For this review, use the dimensioned drawing (mm, ordinates from the lowest corner) and the shaded views. A direction names the side the tool comes from. Give positions to 0.01 mm unless a question says otherwise; leave off trailing zeros. Write each loop counter-clockwise with the first axis right and the second up, starting at its lowest first coordinate (ties: lowest second). Pieces come first, ordered by that corner, then holes. Notation, with made-up numbers: M 45.25,76 L 55.25,76 A22 ccw 55.25,95 Z; hole C -1.5,73.25 d6. An arc over 180 degrees is marked long. One line per item, written item: value. Start each with the question number.
Item 1: Tool access review of the marked faces 1 and 2: name each direction out of +Z, -Z, +X, -X, +Y, -Y from which nothing blocks a thin tool from reaching the whole face with its end or side.
Item 2: Mouldability with a two-part tool opening along X and no side actions: class the marked faces 3, 4 and 5 as released by +X, released by -X, zero draft, split by the parting line, or undercut.
Item 3: Consider section D-D, the plane x = 64.5. Write out the cut boundary in (y, z).
Item 4: Consider section B-B, the plane y = 37.5. Write out the cut boundary in (x, z).
Item 5: Consider section C-C, the plane z = 23. Write out the cut boundary in (x, y), and give its area (3 significant figures).
Item 6: Consider section A-A, the plane x = 39. Write out the cut boundary in (y, z), and give its area (3 significant figures).
Item 7: To check wall thickness, follow probe 1 along X at (y, z) = (17, 9); probe 2 along Z at (x, y) = (64.5, 27.1); probe 3 along Y at (x, z) = (53.5, 16). State the ranges of each line that lie inside material, in increasing order.
Item 8: Clearance check with flat-ended pins moving along their axes: pin 1 Ø3.5 at (x, z) = (64.5, 37) entering from +Y; pin 2 Ø5 at (x, z) = (64.5, 9) entering from -Y; pin 3 Ø0.9 at (x, y) = (36.5, 17.5) entering from -Z. State where each tip first meets the part, or that it passes through.
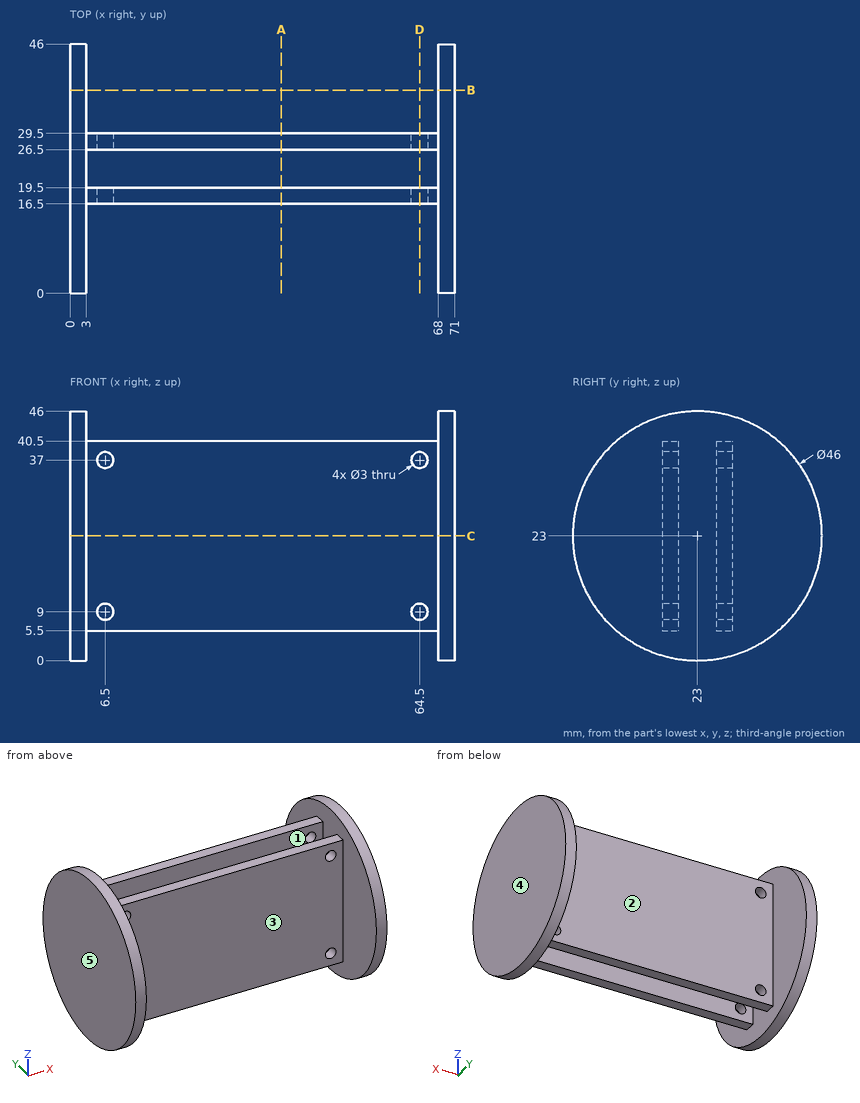
Model answer:
1. face 1: +Z, -Z
1. face 2: +Z, -Z, +Y
2. face 3: undercut
2. face 4: released by +X
2. face 5: released by -X
3. outline: M 16.5,5.5 L 19.5,5.5 L 19.5,7.5 L 16.5,7.5 Z; M 16.5,10.5 L 19.5,10.5 L 19.5,35.5 L 16.5,35.5 Z; M 16.5,38.5 L 19.5,38.5 L 19.5,40.5 L 16.5,40.5 Z; M 26.5,5.5 L 29.5,5.5 L 29.5,7.5 L 26.5,7.5 Z; M 26.5,10.5 L 29.5,10.5 L 29.5,35.5 L 26.5,35.5 Z; M 26.5,38.5 L 29.5,38.5 L 29.5,40.5 L 26.5,40.5 Z
4. outline: M 0,5.15 L 3,5.15 L 3,40.85 L 0,40.85 Z; M 68,5.15 L 71,5.15 L 71,40.85 L 68,40.85 Z
5. outline: M 0,0 L 3,0 L 3,16.5 L 68,16.5 L 68,0 L 71,0 L 71,46 L 68,46 L 68,29.5 L 3,29.5 L 3,46 L 0,46 Z; hole M 3,19.5 L 68,19.5 L 68,26.5 L 3,26.5 Z
5. area: 666 mm2
6. outline: M 16.5,5.5 L 19.5,5.5 L 19.5,40.5 L 16.5,40.5 Z; M 26.5,5.5 L 29.5,5.5 L 29.5,40.5 L 26.5,40.5 Z
6. area: 210 mm2
7. probe 1: x = 0 to 5, 8 to 63, 66 to 71
7. probe 2: z = 5.5 to 7.5, 10.5 to 35.5, 38.5 to 40.5
7. probe 3: y = 16.5 to 19.5, 26.5 to 29.5
8. pin 1: stops at y = 29.5
8. pin 2: stops at y = 16.5
8. pin 3: stops at z = 5.5
